CAD build for the part. Positions are in the model's coordinates, mm. Face numbers are marked on the shaded views. A direction names the side the tool comes from. Round coordinates to 2 decimals unless told otherwise and drop trailing zeros. Loops run counter-clockwise (first coordinate to the right, second up) from the corner with the lowest first, then second, coordinate; pieces in that order, holes last. Notation, with made-up numbers: (80, 42) - (96, 42) arc R35 ccw to (96, 80) - close; hole circle Ø5 at (6.25, 16.25). An arc over 180 degrees is marked (long way). Use one line per item in the form item = value.
from build123d import *

# Parameters (mm, degrees)
SKETCH1_R           = 1
SKETCH1_R_2         = 4
BOSS_EXTRUDE1_DEPTH = 3
SKETCH2_W           = 2.5
SKETCH2_H           = 22
BOSS_EXTRUDE2_DEPTH = 6
SKETCH3_R           = 1
CUT_EXTRUDE1_DEPTH  = 6


with BuildPart() as part:
    # Sketch1 → Boss-Extrude1 (new body)
    with BuildSketch(Plane(origin=(0, 0, 0), x_dir=(1, 0, 0), z_dir=(0, 1, 0))):
        with BuildLine():
            Line((-14, -11), (-14, 11))
            Line((-14, 11), (7, 11))
            ThreePointArc((7, 11), (18, 0), (7, -11))
            Line((7, -11), (-14, -11))
        make_face()
        with Locations((7, -7)):
            Circle(SKETCH1_R, mode=Mode.SUBTRACT)
        Circle(SKETCH1_R, mode=Mode.SUBTRACT)
        with Locations((7, 0)):
            Circle(SKETCH1_R_2, mode=Mode.SUBTRACT)
        with Locations((14, 0)):
            Circle(SKETCH1_R, mode=Mode.SUBTRACT)
        with Locations((7, 7)):
            Circle(SKETCH1_R, mode=Mode.SUBTRACT)
    extrude(amount=BOSS_EXTRUDE1_DEPTH)

    # Sketch2 → Boss-Extrude2 (add)
    with BuildSketch(Plane(origin=(0, 3, 0), x_dir=(1, 0, 0), z_dir=(0, 1, 0))):
        with Locations((-12.75, 0)):
            Rectangle(SKETCH2_W, SKETCH2_H)
    extrude(amount=BOSS_EXTRUDE2_DEPTH)

    # Sketch3 → Cut-Extrude1 (cut)
    with BuildSketch(Plane(origin=(-11.5, 0, 0), x_dir=(0, 0, -1), z_dir=(1, 0, 0))):
        with Locations((8, 6)):
            Circle(SKETCH3_R)
        with Locations((-8, 6)):
            Circle(SKETCH3_R)
    extrude(amount=-CUT_EXTRUDE1_DEPTH, mode=Mode.SUBTRACT)


solid = part.part
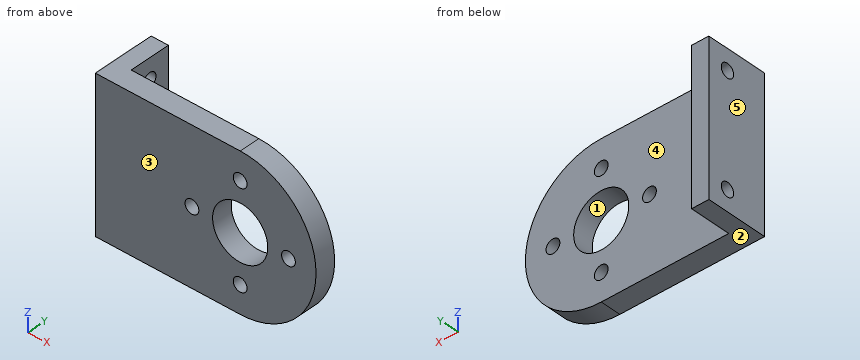
1) Two-plate mould, pull along Z, no slides. Class the marked faces 1, 2 and 3: +Z half, -Z half, draft (parallel to the pull), parting line (faces both ways), or undercut.
Report:
face_1 = undercut
face_2 = -Z half
face_3 = draft
2) Slice it at C-C (x = 14). Write the cut outline in (y, z).
Report:
outline = (0, -8.49) - (3, -8.49) - (3, -1) - (0, -1) - close; (0, 1) - (3, 1) - (3, 8.49) - (0, 8.49) - close
3) Slice it at D-D (y = 2.5). Write the cut outline in (x, z).
Report:
outline = (-14, -11) - (7, -11) arc R11 ccw to (7, 11) - (-14, 11) - close; hole circle Ø2 at (0, 0); hole circle Ø8 at (7, 0); hole circle Ø2 at (7, -7); hole circle Ø2 at (7, 7); hole circle Ø2 at (14, 0)
4) Drill centre lines: probe 1 along X at (y, z) = (1.25, 0); probe 2 along Z at (x, y) = (7, 2); probe 3 along Y at (x, z) = (-2, -8.5). Where is each one in solid material? Low to high.
Report:
probe_1 = -14 to -1, 1 to 3, 11 to 13, 15 to 18
probe_2 = -11 to -8, -6 to -4, 4 to 6, 8 to 11
probe_3 = 0 to 3
5) Slice it at B-B (y = 6). Write the cut outline in (x, z), plus the area to 3 significant figures.
Report:
outline = (-14, -11) - (-11.5, -11) - (-11.5, -9) - (-14, -9) - close; (-14, -7) - (-11.5, -7) - (-11.5, 7) - (-14, 7) - close; (-14, 9) - (-11.5, 9) - (-11.5, 11) - (-14, 11) - close
area = 45.0 mm^2
6) Slice it at A-A (z = 0). Write the cut outline in (x, y), plus the area to 3 significant figures.
Report:
outline = (-14, 0) - (-1, 0) - (-1, 3) - (-11.5, 3) - (-11.5, 9) - (-14, 9) - close; (1, 0) - (3, 0) - (3, 3) - (1, 3) - close; (11, 0) - (13, 0) - (13, 3) - (11, 3) - close; (15, 0) - (18, 0) - (18, 3) - (15, 3) - close
area = 75.0 mm^2
7) Tool access for the marked faces 4 and 5: list every direction of +Z, -Z, +X, -X, +Y, -Y with a clear straight run to the whole face (end or side of a thin tool).
Report:
face_4 = +Z, -Z, +X, +Y
face_5 = +Z, -Z, -X, +Y, -Y
8) Flat gauge pins, fed straight in: pin 1 (1.6 mm diameter, centred on x = 14, z = 0, fed in from -Y); pin 2 (1.8 mm diameter, centred on y = 7.5, z = -0.5, fed in from +X); pin 3 (6 mm diameter, centred on x = 6.5, z = -7, fed in from +Y). Where does each tip first touch, or does it go through?
Report:
pin_1 = through
pin_2 = -11.5
pin_3 = 3
